Input: dimensioned drawing with shaded views. Units: mm. Origin: part minimum x, y, z. Give positions to 0.01 mm unless a question says otherwise; leave off trailing zeros. Write each loop counter-clockwise with the first axis right and the second up, starting at its lowest first coordinate (ties: lowest second). Pieces come first, ordered by that corner, then holes. Notation, with made-up numbers: (17.5, -6) -> (26.5, -6) arc R9 cw to (26.5, 9) -> close; hole circle Ø11 at (66, 50). An arc over 180 degrees is marked (long way). Return JSON: item names as keys, results as strings. Group by question number.
Item 1: Section A-A, the plane y = 1.27. Return loops of the section in (x, z).
Item 2: Section D-D, the plane y = 2.25. Return loops of the section in (x, z).
Item 3: Pin query (flat end, axial travel): P1, Ø1.5, axis at y = 2, z = 7, coming from the -X side. Return the tip coordinate at first contact, or that it passes through.
Item 4: Section B-B, the plane x = 3.81. Return loops of the section in (y, z).
Item 5: Line query: line 1 (Y direction, x = 3.81, z = 7.75); line 2 (X direction, y = 1.2, z = 3.25); line 3 (X direction, y = 1.6, z = 5.75). Output: solid intervals per line, ascending. Write a range as [from, to].
Item 6: Section C-C, the plane z = 4. Return loops of the section in (x, y), then the cut area to 3 significant figures.
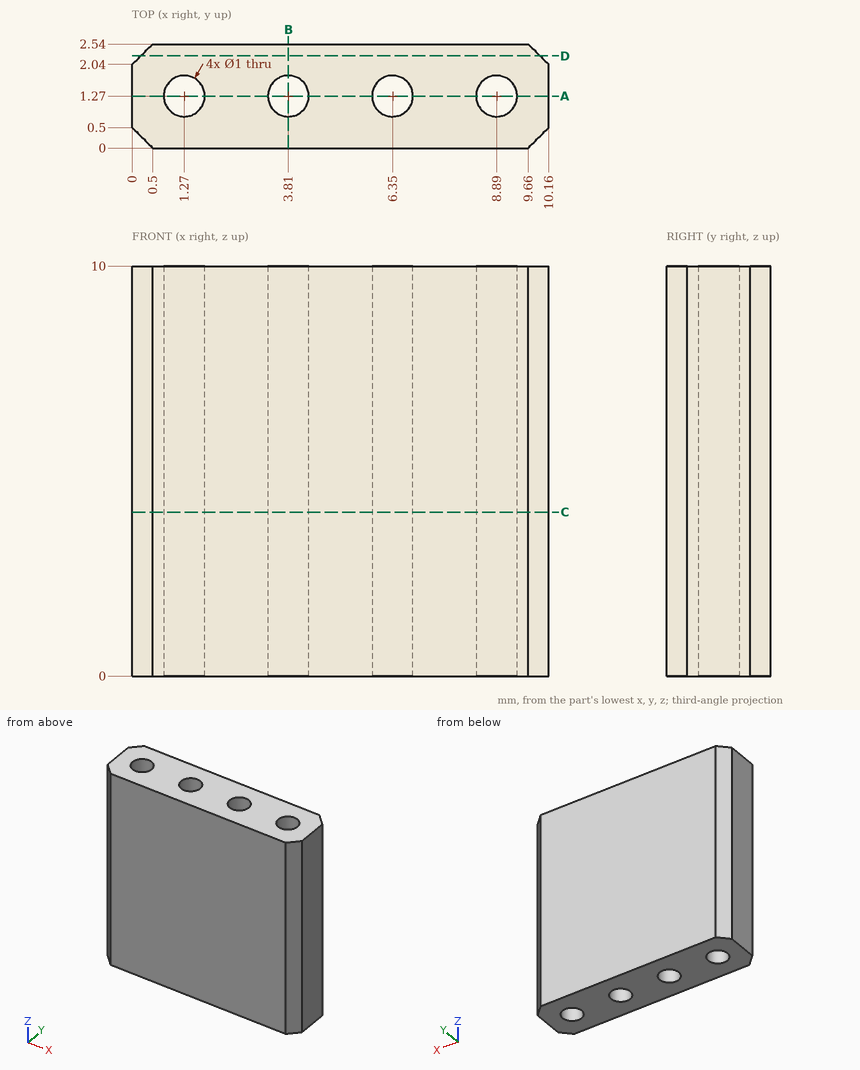
Answer below:
{
 "1": {"outline": "(0, 0) -> (0.77, 0) -> (0.77, 10) -> (0, 10) -> close; (1.77, 0) -> (3.31, 0) -> (3.31, 10) -> (1.77, 10) -> close; (4.31, 0) -> (5.85, 0) -> (5.85, 10) -> (4.31, 10) -> close; (6.85, 0) -> (8.39, 0) -> (8.39, 10) -> (6.85, 10) -> close; (9.39, 0) -> (10.16, 0) -> (10.16, 10) -> (9.39, 10) -> close"},
 "2": {"outline": "(0.21, 0) -> (9.95, 0) -> (9.95, 10) -> (0.21, 10) -> close"},
 "3": {"P1": "stops at x = 0"},
 "4": {"outline": "(0, 0) -> (0.77, 0) -> (0.77, 10) -> (0, 10) -> close; (1.77, 0) -> (2.54, 0) -> (2.54, 10) -> (1.77, 10) -> close"},
 "5": {"line 1": "y = [0, 0.77], [1.77, 2.54]", "line 2": "x = [0, 0.77], [1.77, 3.31], [4.31, 5.85], [6.85, 8.39], [9.39, 10.16]", "line 3": "x = [0, 0.89], [1.65, 3.43], [4.19, 5.97], [6.73, 8.51], [9.27, 10.16]"},
 "6": {"outline": "(0, 0.5) -> (0.5, 0) -> (9.66, 0) -> (10.16, 0.5) -> (10.16, 2.04) -> (9.66, 2.54) -> (0.5, 2.54) -> (0, 2.04) -> close; hole circle Ø1 at (1.27, 1.27); hole circle Ø1 at (3.81, 1.27); hole circle Ø1 at (6.35, 1.27); hole circle Ø1 at (8.89, 1.27)", "area": "22.2 mm2"}
}
